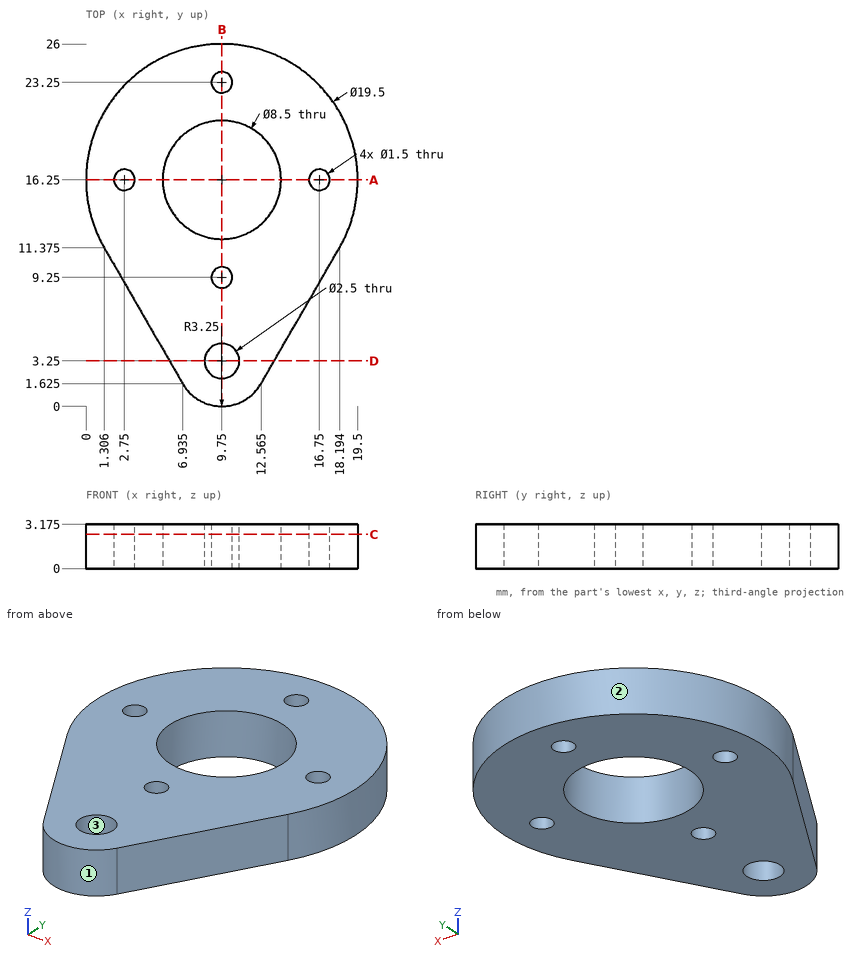
Could you check a few things on this drawing? It's one solid part, dimensions in mm from its lowest x, y, z. Give positions to 0.01 mm unless a question says otherwise; leave off trailing zeros. Write each loop counter-clockwise with the first axis right and the second up, starting at its lowest first coordinate (ties: lowest second). Pieces come first, ordered by that corner, then holes. Notation, with made-up numbers: (-17.5, -22) -> (7.5, -22) arc R20 cw to (7.5, -6) -> close; hole circle Ø4 at (57.25, 39.5). An arc over 180 degrees is marked (long way). Write item = value, one per line.
(1) I'm going to push a flat-ended pin straight in: P1, Ø1.4, axis at x = 9.75, y = 9.25, coming from the -Z side. Where does the tip first touch, or does it pass through?
Worked out:
P1 = through
(2) Suppose I cut it at A-A on y = 16.25. Write out the boundary of the cut face in (x, z) (1 decimal).
Worked out:
outline = (0, 0) -> (2, 0) -> (2, 3.2) -> (0, 3.2) -> close; (3.5, 0) -> (5.5, 0) -> (5.5, 3.2) -> (3.5, 3.2) -> close; (14, 0) -> (16, 0) -> (16, 3.2) -> (14, 3.2) -> close; (17.5, 0) -> (19.5, 0) -> (19.5, 3.2) -> (17.5, 3.2) -> close
(3) Suppose I cut it at D-D on y = 3.25. Write out the boundary of the cut face in (x, z) (1 decimal).
Worked out:
outline = (6, 0) -> (8.5, 0) -> (8.5, 3.2) -> (6, 3.2) -> close; (11, 0) -> (13.5, 0) -> (13.5, 3.2) -> (11, 3.2) -> close
(4) I need wall thicknesses on probe 1 along X at (y, z) = (16.5, 2.6); probe 2 along Y at (x, z) = (16.75, 2.35) (1 decimal); probe 3 along Y at (x, z) = (6.5, 2.3) (1 decimal). Which ranges of each line are inside material? Lowest first, please. Write a range as from..to.
Worked out:
probe_1 = 0..2.04, 3.46..5.51, 13.99..16.04, 17.46..19.5
probe_2 = 8.9..15.5, 17..23
probe_3 = 2.4..13.5, 19..25.4
(5) Suppose I cut it at C-C on z = 2.45. Count the separate pieces of the cut face and the enclosed holes in it, then the cut area to 3 significant figures.
Worked out:
separate_pieces = 1
enclosed_holes = 6
area = 288 mm^2
(6) Thinking about a two-plate mould opening in Y: for the marked faces 1, 2 and 3, which applies, released by +Y, released by -Y, zero draft, split by the parting line, or undercut?
Worked out:
face_1 = released by -Y
face_2 = split by the parting line
face_3 = undercut
(7) Suppose I cut it at B-B on x = 9.75. Write out the boundary of the cut face in (y, z) (1 decimal), then the cut area to 3 significant figures.
Worked out:
outline = (0, 0) -> (2, 0) -> (2, 3.2) -> (0, 3.2) -> close; (4.5, 0) -> (8.5, 0) -> (8.5, 3.2) -> (4.5, 3.2) -> close; (10, 0) -> (12, 0) -> (12, 3.2) -> (10, 3.2) -> close; (20.5, 0) -> (22.5, 0) -> (22.5, 3.2) -> (20.5, 3.2) -> close; (24, 0) -> (26, 0) -> (26, 3.2) -> (24, 3.2) -> close
area = 38.1 mm^2
